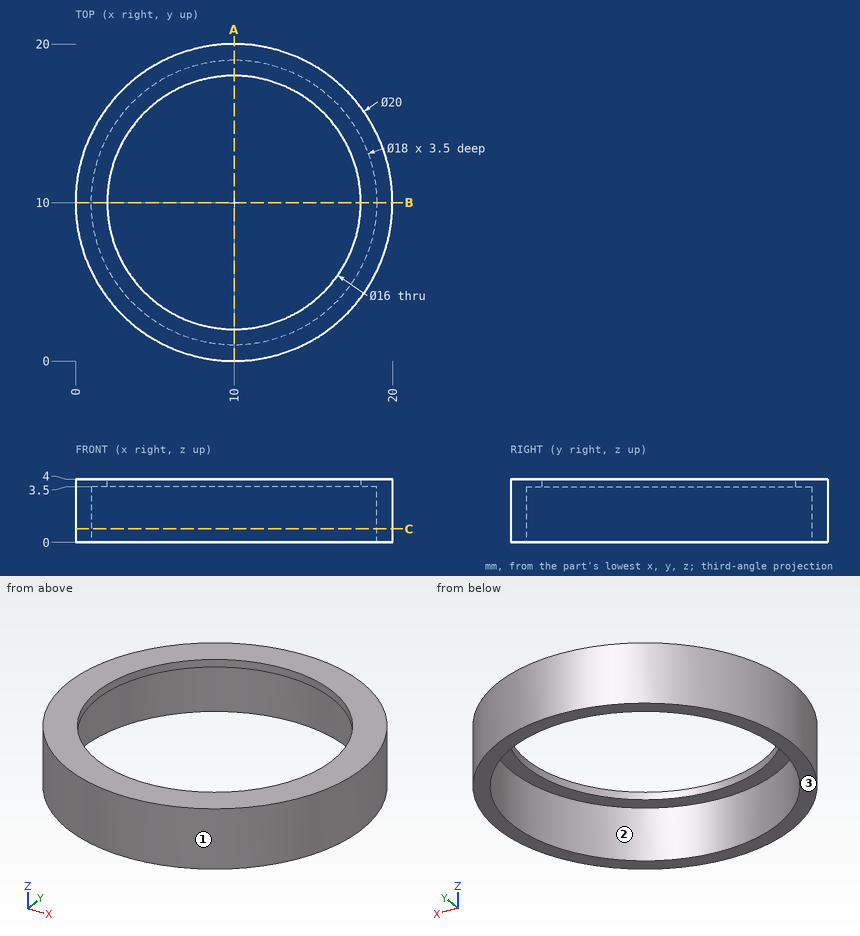
Print and shaded views of the part. All mm, measured from the part's lowest x, y and z. Coordinates: 2 decimals unless noted, no trailing zeros. Write each loop counter-clockwise with the first axis right and the second up, starting at its lowest first coordinate (ties: lowest second). Pieces come first, ordered by that corner, then holes.
(1) Drill centre lines: probe 1 along Y at (x, z) = (10, 3.85); probe 2 along Y at (x, z) = (10, 1.35); probe 3 along X at (y, z) = (8.25, 1.25). Where is each one in solid material? Low to high.
(2) Cut at A-A, the plane x = 10. List the corners of the cut face in (y, z).
(3) Flat gauge pins, fed straight in: pin 1 (6 mm diameter, centred on x = 6.5, y = 14, fed in from -Z); pin 2 (6 mm diameter, centred on x = 7.5, y = 14.5, fed in from +Z). Where does each tip first touch, or does it go through?
(4) Two-plate mould, pull along Y, no slides. Class the marked faces 1, 2 and 3: +Y half, -Y half, draft (parallel to the pull), parting line (faces both ways), or undercut.
(5) Cut at C-C, the plane z = 0.85. List the corners of the cut face in (x, y).
Geometry says:
1. probe 1: y = 0 to 2, 18 to 20
1. probe 2: y = 0 to 1, 19 to 20
1. probe 3: x = 0.15 to 1.17, 18.83 to 19.85
2. outline: (0, 0) - (1, 0) - (1, 3.5) - (2, 3.5) - (2, 4) - (0, 4) - close; (18, 3.5) - (19, 3.5) - (19, 0) - (20, 0) - (20, 4) - (18, 4) - close
3. pin 1: stops at z = 3.5
3. pin 2: stops at z = 4
4. face 1: parting line
4. face 2: undercut
4. face 3: draft
5. outline: circle Ø20 at (10, 10); hole circle Ø18 at (10, 10)
